Could you check a few things on this model? Use its own coordinates, in mm. A direction names the side the tool comes from. Round coordinates to 2 decimals unless told otherwise and drop trailing zeros. Loops run counter-clockwise (first coordinate to the right, second up) from the corner with the lowest first, then second, coordinate; pieces in that order, holes last. Notation, with made-up numbers: (52, 1) - (68, 1) arc R35 cw to (68, 38) - close; hole circle Ø4 at (48.5, -17). An arc over 180 degrees is marked (long way). Answer as CSV lines item,"result". Start each with the question number.
1) Which directions (+Z, -Z, +X, -X, +Y, -Y) give clear straight access to the entire face, cutting with the end or side of a thin tool? Please do faces 1 (the face through (-1.172, 8.923, 2.26)), 2 (the face through (18.71, -10.57, 1.48)).
2) Suppose I cut it at C-C, the plane x = 4. Write out the boundary of the cut face in (y, z), then the cut area to 3 significant figures.
3) Suppose I cut it at A-A, the plane y = -20. Write out the boundary of the cut face in (x, z).
4) We'd pull the mould along X, two halves only. Please class faces 3 (the face through (-4.68, -2.49, 1.52)), 4 (the face through (-0.3, 11.5, 3)), 5 (the face through (23.846, 7.509, 1.479)): pulls with the +X half, pulls with the -X half, needs draft (parallel to the pull), parting line crosses it, or undercut.
5) Please list where these lines run through material, in increasing order: line 1 along Y through (x, z) = (0, 2.25); line 2 along Y through (x, z) = (1, 1.55); line 3 along Y through (x, z) = (-8, 1.9).
6) Suppose I cut it at B-B, the plane z = 2.1. Count the separate pieces of the cut face and the enclosed holes in it, then the cut area to 3 significant figures.
7) I'm going to push flat-ended pins straight in: pin 1 Ø1.5 at (y, z) = (-14.5, 1) entering from +X; pin 2 Ø1.5 at (x, z) = (-19, 0.5) entering from -Y. Where does each tip first touch, or does it pass through?
8) Suppose I cut it at D-D, the plane y = -10. Write out the boundary of the cut face in (x, z).
```python
from build123d import *

# Parameters (mm, degrees)
SKETCH_1_R          = 25
SKETCH_1_R_2        = 2.5
SKETCH_1_R_3        = 1.65
SKETCH_1_R_4        = 1.5
SKETCH_1_R_5        = 11.05
EXTRUDE_1_DEPTH     = 3
SKETCH_2_R          = 11.15
SKETCH_2_R_2        = 9
CUT_EXTRUDE_1_DEPTH = 1.5
SKETCH_4_R          = 1.55
CUT_EXTRUDE_2_DEPTH = 36.482389998


with BuildPart() as part:
    # 草图1 → 凸台-拉伸1 (new body)
    # profile 1 of 2: a face of its own
    with BuildSketch(Plane.XY):
        Circle(SKETCH_1_R)
        with Locations((0, -20)):
            Circle(SKETCH_1_R_2, mode=Mode.SUBTRACT)
        with Locations((0, 20)):
            Circle(SKETCH_1_R_3, mode=Mode.SUBTRACT)
        with Locations((-17.320508076, -10)):
            Circle(SKETCH_1_R_3, mode=Mode.SUBTRACT)
        with Locations((17.320508076, -10)):
            Circle(SKETCH_1_R_4, mode=Mode.SUBTRACT)
        Circle(SKETCH_1_R_5, mode=Mode.SUBTRACT)
    # profile 2 of 2: a face of its own
    with BuildSketch(Plane.XY):
        Circle(SKETCH_1_R_5)
    extrude(amount=EXTRUDE_1_DEPTH)

    # 草图2 → 切除-拉伸1 (cut)
    with BuildSketch(Plane.XY.offset(3)):
        Circle(SKETCH_2_R)
        Circle(SKETCH_2_R_2, mode=Mode.SUBTRACT)
    extrude(amount=-CUT_EXTRUDE_1_DEPTH, mode=Mode.SUBTRACT)

    # 草图4 → 切除-拉伸2 (cut, through all)
    with BuildSketch(Plane.XY.offset(3)):
        with Locations((-3.535533906, 3.535533906)):
            Circle(SKETCH_4_R)
        with Locations((3.535533906, 3.535533906)):
            Circle(SKETCH_4_R)
        with Locations((3.535533906, -3.535533906)):
            Circle(SKETCH_4_R)
        with Locations((-3.535533906, -3.535533906)):
            Circle(SKETCH_4_R)
    extrude(amount=-CUT_EXTRUDE_2_DEPTH, mode=Mode.SUBTRACT)


solid = part.part
```
Filled sheet:
1,face 1,"+Z"
1,face 2,"+Z, -Z"
2,outline,"(-24.68, 0) - (-5.01, 0) - (-5.01, 3) - (-8.06, 3) - (-8.06, 1.5) - (-10.41, 1.5) - (-10.41, 3) - (-24.68, 3) - close; (-2.06, 0) - (2.06, 0) - (2.06, 3) - (-2.06, 3) - close; (5.01, 0) - (24.68, 0) - (24.68, 3) - (10.41, 3) - (10.41, 1.5) - (8.06, 1.5) - (8.06, 3) - (5.01, 3) - close"
2,area,"123 mm²"
3,outline,"(-15, 0) - (-2.5, 0) - (-2.5, 3) - (-15, 3) - close; (2.5, 0) - (15, 0) - (15, 3) - (2.5, 3) - close"
4,face 3,"undercut"
4,face 4,"needs draft"
4,face 5,"parting line crosses it"
5,line 1,"-25 to -22.5, -17.5 to -11.15, -9 to 9, 11.15 to 18.35, 21.65 to 25"
5,line 2,"-24.98 to -22.29, -17.71 to -11.11, -8.94 to 8.94, 11.11 to 18.69, 21.31 to 24.98"
5,line 3,"-23.69 to -7.77, -4.12 to 4.12, 7.77 to 23.69"
6,separate pieces,"2"
6,enclosed holes,"9"
6,area,"1,750 mm²"
7,pin 1,"x = 20.88"
7,pin 2,"y = -17.09"
8,outline,"(-22.91, 0) - (-18.97, 0) - (-18.97, 3) - (-22.91, 3) - close; (-15.67, 0) - (15.82, 0) - (15.82, 3) - (4.93, 3) - (4.93, 1.5) - (-4.93, 1.5) - (-4.93, 3) - (-15.67, 3) - close; (18.82, 0) - (22.91, 0) - (22.91, 3) - (18.82, 3) - close"
